Check sheet for the modelled part. Datum: model origin and axes. Units: mm. A direction names the side the tool comes from. Coordinates: 2 decimals unless noted, no trailing zeros. Write each loop counter-clockwise with the first axis right and the second up, starting at its lowest first coordinate (ties: lowest second). Pieces come first, ordered by that corner, then holes. Notation, with made-up numbers: (44, 7.5) - (77, 7.5) arc R18 ccw to (77, 36.5) - close; hole circle Ø1 at (-19.75, 24). An arc over 180 degrees is marked (long way). Write each question's results on one line, items separated by ' | '.
Autodesk Inventor part; units mm, degrees
ref_plane "Work Plane4" through (-54.4, 1.6, -9.4) normal (1, 0, 0) x (0, 0, -1)
ref_plane "YZ Plane" through (0, 0, 0) normal (1, 0, 0) x (0, 1, 0)
ref_plane "XZ Plane" through (0, 0, 0) normal (0, 1, 0) x (-1, 0, 0)
sketch "Sketch1" plane through (0, 0, 0) normal (0, 1, 0) x (-1, 0, 0)
  line L0 (0, 0) -> (100, 0)
  line L1 (100, 0) -> (100, -80)
  line L2 (100, -80) -> (0, -80)
  line L3 (0, -80) -> (0, 0)
  dimension "d0" = 100
  dimension "d1" = 80
extrude "LidBase" add sketch "Sketch1" along normal blind 1.6
fillet "Fillet1" radius 5 4 edges at (-100, 0.8, 0) (0, 0.8, 0) (0, 0.8, -80) (-100, 0.8, -80)
sketch "Sketch3" plane through (0, 1.6, 0) normal (0, 1, 0) x (1, 0, 0)
  line L0 (-5, 80) -> (-95, 80)
  arc A0 (-95, 80) -> (-100, 75) centre (-95, 75) ccw
  line L1 (-100, 75) -> (-100, 5)
  arc A1 (-100, 5) -> (-95, 0) centre (-95, 5) ccw
  line L2 (-95, 0) -> (-5, 0)
  arc A2 (-5, 0) -> (0, 5) centre (-5, 5) ccw
  line L3 (0, 5) -> (0, 75)
  arc A3 (0, 75) -> (-5, 80) centre (-5, 75) ccw
  line L4 (-5, 80) -> (-95, 80)
  line L5 (-95.6, 75.6) -> (-4.4, 75.6)
  line L6 (-4.4, 75.6) -> (-4.4, 4.4)
  line L7 (-4.4, 4.4) -> (-95.6, 4.4)
  line L8 (-95.6, 4.4) -> (-95.6, 75.6)
  point P0 (0, 0)
  dimension "d5" = 4.4
  dimension "d6" = 4.4
  dimension "d7" = 4.4
  dimension "d8" = 4.4
extrude "Gasket Seal" add sketch "Sketch3" along normal blind 5 contours L5 L6 L7 L8
fillet "Fillet2" radius 5 4 edges at (-4.4, 4.1, -4.4) (-4.4, 4.1, -75.6) (-95.6, 4.1, -75.6) (-95.6, 4.1, -4.4)
ref_plane "Work Plane4" through (-54.4, 1.6, -9.4) normal (1, 0, 0) x (0, 0, -1)
sketch "Sketch7" plane through (-54.4, 1.6, -9.4) normal (1, 0, 0) x (0, 0, -1)
  line L0 (70.6, -1.6) -> (-9.4, -1.6)
  line L1 (-9.4, -1.6) -> (-9.4, 0)
  line L2 (-9.4, 0) -> (-5, 0)
  line L3 (-5, 0) -> (-5, 5)
  line L4 (-5, 5) -> (66.2, 5)
  line L5 (66.2, 5) -> (66.2, 0)
  line L6 (66.2, 0) -> (70.6, 0)
  line L7 (70.6, 0) -> (70.6, -1.6)
  circle A0 centre (-6, 2.5) radius 1.8
  point P0 (-9.4, -1.6)
  dimension "d24" = 3.6
  dimension "d25" = 2.5
  dimension "d26" = 1
sketch3d "3D Sketch3"
  line L0 (-90.6, 1.6, -4.4) -> (-9.4, 1.6, -4.4)
  arc A0 (-9.4, 1.6, -4.4) -> (-4.4, 1.6, -9.4) centre (-9.4, 1.6, -9.4) ccw
  line L1 (-4.4, 1.6, -9.4) -> (-4.4, 1.6, -70.6)
  arc A1 (-4.4, 1.6, -70.6) -> (-9.4, 1.6, -75.6) centre (-9.4, 1.6, -70.6) ccw
  line L2 (-9.4, 1.6, -75.6) -> (-90.6, 1.6, -75.6)
  arc A2 (-90.6, 1.6, -75.6) -> (-95.6, 1.6, -70.6) centre (-90.6, 1.6, -70.6) ccw
  line L3 (-95.6, 1.6, -70.6) -> (-95.6, 1.6, -9.4)
  arc A3 (-95.6, 1.6, -9.4) -> (-90.6, 1.6, -4.4) centre (-90.6, 1.6, -9.4) ccw
sweep "Oring Channel" cut profiles "Sketch7" path "3D Sketch3" contours A0 L3 | L3 A0
sketch "Sketch8" plane through (0, 0, 0) normal (0, 1, 0) x (1, 0, 0)
  line L0 (-100, 75) -> (-100, 5)
  line L1 (-95, 0) -> (-5, 0)
  line L2 (-9.4, 75.6) -> (-90.6, 75.6)
  line L3 (-5, 80) -> (-95, 80)
  line L4 (0, 5) -> (0, 75)
  point P0 (0, 0)
  point P1 (-80.2, 9.8)
  point P2 (-19.8, 9.8)
  point P3 (-19.8, 70.2)
  point P4 (-80.2, 70.2)
  dimension "d29" = 19.8
  dimension "d30" = 9.8
  dimension "d32" = 9.8
  dimension "d33" = 19.8
  dimension "d34" = 19.8
  dimension "d35" = 9.8
  dimension "d36" = 19.8
  dimension "d37" = 9.8
hole "Hole1" at (-80.2, 0, -9.8) at (-19.8, 0, -9.8) at (-19.8, 0, -70.2) at (-80.2, 0, -70.2) direction (0, 1, 0) diameter 4.4 end through all counterbore diameter 8.2 counterbore depth 3.2
equation "\"d6\" = d5"
equation "\"d7\" = d5"
equation "\"d8\" = d5"
properties part number "Lid"
1. Sectioned sample at B-B (x = -48). Record the cut outline in (y, z).
Values follow:
outline: (0, -80) - (1.6, -80) - (1.6, -75.6) - (2.6, -75.6) arc R1.8 cw to (5.6, -75.6) - (6.6, -75.6) - (6.6, -4.4) - (5.6, -4.4) arc R1.8 cw to (2.6, -4.4) - (1.6, -4.4) - (1.6, 0) - (0, 0) - close
2. Access from +Z, -Z, +X, -X, +Y, -Y to the whole of each face (thin tool, end or side, straight path). Record for faces 4 (the cylindrical face through (-94.1, 2.11, -74.17)), 5 (the cylindrical face through (-5.9, 6.11, -5.83)), 6 (the flat face through (-39, 1.6, -4)), 7 (the cylindrical face through (-5.83, 6.11, -74.1)), 8 (the cylindrical face through (-19.98, 1.622, -66.104)).
Values follow:
face 4: -Z, -X, +Y | face 5: +Z, +X, +Y | face 6: +Y | face 7: -Z, +X, +Y | face 8: -Y
3. Sectioned sample at A-A (x = -80.2). Record the cut outline in (y, z), then the cut area to 3 significant figures.
Values follow:
outline: (0, -80) - (1.6, -80) - (1.6, -75.6) - (2.6, -75.6) arc R1.8 cw to (5.6, -75.6) - (6.6, -75.6) - (6.6, -72.4) - (3.2, -72.4) - (3.2, -74.3) - (0, -74.3) - close; (0, -66.1) - (3.2, -66.1) - (3.2, -68) - (6.6, -68) - (6.6, -12) - (3.2, -12) - (3.2, -13.9) - (0, -13.9) - close; (0, -5.7) - (3.2, -5.7) - (3.2, -7.6) - (6.6, -7.6) - (6.6, -4.4) - (5.6, -4.4) arc R1.8 cw to (2.6, -4.4) - (1.6, -4.4) - (1.6, 0) - (0, 0) - close | area: 398 mm^2
4. Sectioned sample at C-C (y = 4.5). Record the cut outline in (x, z) (3 decimals).
Values follow:
outline: (-94.845, -70.6) arc R4.245 ccw to (-90.6, -74.845) - (-9.4, -74.845) arc R4.245 ccw to (-5.155, -70.6) - (-5.155, -9.4) arc R4.245 ccw to (-9.4, -5.155) - (-90.6, -5.155) arc R4.245 ccw to (-94.845, -9.4) - close; hole circle Ø4.4 at (-80.2, -70.2); hole circle Ø4.4 at (-80.2, -9.8); hole circle Ø4.4 at (-19.8, -70.2); hole circle Ø4.4 at (-19.8, -9.8)
5. Material ranges on L1, parallel to Z at x = -19.8, y = 1.35; L2, parallel to X at y = 5.8, z = -9.8; L3, parallel to X at y = 4.4, z = -70.2, recorded low to high. Write a range as [from, to].
Values follow:
L1: z = [-80, -74.3], [-66.1, -13.9], [-5.7, 0] | L2: x = [-95.6, -82.4], [-78, -22], [-17.6, -4.4] | L3: x = [-94.83, -82.4], [-78, -22], [-17.6, -5.17]
6. Draft check along Z on faces 1 (the cylindrical face through (-98, 1, -79)), 2 (the cylindrical face through (-5.9, 2.11, -5.83)), 3 (the flat face through (-18, 3.2, -12)). Enter one of: pulls with the +Z half, pulls with the -Z half, needs draft (parallel to the pull), parting line crosses it, or undercut.
Values follow:
face 1: pulls with the -Z half | face 2: pulls with the +Z half | face 3: undercut
7. Go/stop test with flat-tipped pins: pin 1 (6.5 mm diameter, centred on x = -19.8, z = -9.8, fed in from -Y); pin 2 (0.5 mm diameter, centred on x = -31, y = 2, fed in from +Z); pin 3 (1 mm diameter, centred on x = -42.5, y = 2.5, fed in from -Z). Record where each tip stops, or that it passes through.
Values follow:
pin 1: stops at y = 3.2 | pin 2: stops at z = -4.4 | pin 3: stops at z = -75.6
